The listing builds one solid part. Answer for the finished solid, in the listing's coordinates (mm). A direction names the side the tool comes from. Give positions to 0.01 mm unless a question says otherwise; leave off trailing zeros. Loops run counter-clockwise (first coordinate to the right, second up) from the corner with the lowest first, then second, coordinate; pieces in that order, holes last. Notation, with made-up numbers: (-30, -20) - (-9, -20) arc R25 cw to (-9, 13) - close; hole circle Ø6 at (-28, 44). An arc over 180 degrees is marked (long way). Write each question's results on one line, items separated by ' | '.
from build123d import *

# Parameters (mm, degrees)
F0_R           = 45
F1_DEPTH       = 10
F2_R           = 15
F3_DEPTH       = 250
F5_D           = 5
F5_CSINK_D     = 10
F5_CSINK_ANGLE = 90
F6_R           = 7
F7_R           = 2
F8_R           = 2
F10_R          = 10
F11_DEPTH      = 230


with BuildPart() as f1:
    # F0 (on Top) → F1 (new body)
    with BuildSketch(Plane.XY):
        Circle(F0_R)
    extrude(amount=F1_DEPTH)

    # F2 (on Top) → F3 (join)
    with BuildSketch(Plane.XY):
        Circle(F2_R)
    extrude(amount=F3_DEPTH)

    # F5 (through all)
    with Locations(Plane.XY.offset(10)):
        with Locations((0, 35), (-30.310889, 17.5), (-30.310889, -17.5), (0, -35), (30.310889, -17.5), (30.310889, 17.5)):
            CounterSinkHole(F5_D / 2, F5_CSINK_D / 2, counter_sink_angle=F5_CSINK_ANGLE)

    # F6
    f6_edges = [f1.edges().sort_by_distance(p)[0] for p in [
        (-15, 0, 10),
    ]]
    fillet(f6_edges, radius=F6_R)

    # F7
    f7_edges = [f1.edges().sort_by_distance(p)[0] for p in [
        (-15, 0, 250),
    ]]
    fillet(f7_edges, radius=F7_R)

    # F8
    f8_edges = [f1.edges().sort_by_distance(p)[0] for p in [
        (-45, 0, 10),
    ]]
    fillet(f8_edges, radius=F8_R)

    # F10 (on face) → F11 (cut)
    with BuildSketch(Plane.XY.offset(250)):
        Circle(F10_R)
    extrude(amount=-F11_DEPTH, mode=Mode.SUBTRACT)


solid = f1.part
Item 1: For faces 1 (the face through (-2.17, -9.76, 136.61)), 2 (the face through (-1, 1, 0)), determine the directions among +Z, -Z, +X, -X, +Y, -Y from which every point of the face is accessible in a straight line to the end or side of a thin tool.
Values found:
face 1: +Z | face 2: -Z, +X, -X, +Y, -Y
Item 2: A cutting plane is placed at B-B, the plane y = 0. Determine the outline of the cut face in (x, z).
Values found:
outline: (-45, 0) - (45, 0) - (45, 8) arc R2 ccw to (43, 10) - (22, 10) arc R7 cw to (15, 17) - (15, 248) arc R2 ccw to (13, 250) - (10, 250) - (10, 20) - (-10, 20) - (-10, 250) - (-13, 250) arc R2 ccw to (-15, 248) - (-15, 17) arc R7 cw to (-22, 10) - (-43, 10) arc R2 ccw to (-45, 8) - close
Item 3: Flat-ended cylindrical pins translate along their axes: P1, Ø8, axis at x = 32, y = 14, coming from the -Z side; P2, Ø1.5, axis at x = -29, y = -32.5, coming from the +Z side; P3, Ø3, axis at x = 0, y = -35, coming from the +Z side; P4, Ø6.5, axis at x = -30.31, y = -17.5, coming from the +Z side. Find the tip coordinate at first contact, or state that the pin passes through.
Values found:
P1: stops at z = 0 | P2: stops at z = 10 | P3: passes through | P4: stops at z = 8.25
Item 4: A cutting plane is placed at A-A, the plane x = 0. Count the separate pieces of the cut face and the enclosed holes in it, plus the area to 3 significant figures.
Values found:
separate pieces: 3 | enclosed holes: 0 | area: 3,410 mm²
Item 5: A cutting plane is placed at C-C, the plane z = 215.5. Determine the outline of the cut face in (x, y).
Values found:
outline: circle Ø30 at (0, 0); hole circle Ø20 at (0, 0)
Item 6: Find the intervals of material crossed by line 1 along Y through (x, z) = (0, 4); line 2 along Y through (x, z) = (8, 108); line 3 along Z through (x, y) = (40.5, -13.5), in increasing order. Write a range as [from, to].
Values found:
line 1: y = [-45, -37.5], [-32.5, 32.5], [37.5, 45] | line 2: y = [-12.69, -6], [6, 12.69] | line 3: z = [0, 10]
Item 7: For a pull along Y with two mould halves and no side action, classify faces 3 (the face through (7, -8, 250)), 4 (the face through (-14.985, 0.66, 130.883)), 5 (the face through (28.002, -18.458, 3.698)) as released by +Y, released by -Y, zero draft, split by the parting line, or undercut.
Values found:
face 3: zero draft | face 4: split by the parting line | face 5: undercut
